Solid Edge part; units mm, degrees
sketch "Sketch1" plane through (0, 0, 0) normal (0, 0, 1) x (1, 0, 0)
  line L0 (-22.225, -31.115) -> (37.465, -31.115)
  line L1 (37.465, -31.115) -> (37.465, 31.115)
  line L2 (-37.465, 31.115) -> (37.465, 31.115)
  line L3 (-37.465, -12.065) -> (-37.465, 31.115)
  line L4 (-37.465, -12.065) -> (-22.225, -27.305)
  line L5 (-22.225, -27.305) -> (-22.225, -31.115)
  circle A0 centre (-26.035, -16.03) radius 1.5625
  circle A1 centre (-32.385, 27.15) radius 1.5625
  circle A2 centre (32.385, 6.83) radius 1.5625
extrude "Protrusion1" add sketch "Sketch1" along normal blind 1.5
sketch "Sketch2" plane through (0, 0, 1.5) normal (0, 0, 1) x (1, 0, 0)
  line L0 (4.1366, -24.673) -> (4.1366, 20.327)
  line L1 (4.1366, 20.327) -> (-13.8634, 20.327)
  line L2 (-13.8634, 20.327) -> (-13.8634, -24.673)
  line L3 (-13.8634, -24.673) -> (4.1366, -24.673)
extrude "ExtrudedProtrusion_2" add sketch "Sketch2" along normal blind 18
sketch "Sketch3" plane through (-4.8634, -24.673, 10.5) normal (0, -1, 0) x (1, 0, 0)
  line L0 (-7.5, -9) -> (-7.5, 6.914)
  line L1 (-7.5, 6.914) -> (7.5, 6.914)
  line L2 (7.5, 6.914) -> (7.5, -9)
  line L3 (7.5, -9) -> (-7.5, -9)
extrude "ExtrudedCutout_1" cut sketch "Sketch3" against normal blind 56
sketch "Sketch4" plane through (-4.8634, -24.673, 10.5) normal (0, -1, 0) x (1, 0, 0)
  line L0 (10, 6.914) -> (-10, 6.914)
  line L1 (-10, 6.914) -> (-10, 9)
  line L2 (-10, 9) -> (10, 9)
  line L3 (10, 9) -> (10, 6.914)
extrude "ExtrudedProtrusion_3" add sketch "Sketch4" against normal blind 45
sketch "Sketch5" plane through (-4.8634, 20.327, 10.5) normal (0, 1, 0) x (-1, 0, 0)
  line L0 (3.5, 12.5) -> (-3.5, 12.5)
  arc A0 (-3.5, 12.5) -> (-4, 12) centre (-3.5, 12) ccw
  line L1 (-4, 12) -> (-4, 11)
  arc A1 (-4, 11) -> (-3.5, 10.5) centre (-3.5, 11) ccw
  arc A2 (-3.5, 10.5) -> (-3, 10) centre (-3.5, 10) cw
  line L2 (-3, 10) -> (-3, 9.5)
  arc A3 (-3, 9.5) -> (-2.5, 9) centre (-2.5, 9.5) ccw
  line L3 (-2.5, 9) -> (2.5, 9)
  arc A4 (2.5, 9) -> (3, 9.5) centre (2.5, 9.5) ccw
  line L4 (3, 9.5) -> (3, 10)
  arc A5 (3, 10) -> (3.5, 10.5) centre (3.5, 10) cw
  arc A6 (4, 11) -> (3.5, 10.5) centre (3.5, 11) cw
  line L5 (4, 11) -> (4, 12)
  arc A7 (3.5, 12.5) -> (4, 12) centre (3.5, 12) cw
extrude "ExtrudedProtrusion_4" add sketch "Sketch5" along normal mid plane 8
Verification items for the finished model (mm, model axes). A direction names the side the tool comes from. Coordinates: 2 decimals unless noted, no trailing zeros. Loops run counter-clockwise (first coordinate to the right, second up) from the corner with the lowest first, then second, coordinate; pieces in that order, holes last. Notation, with made-up numbers: (42.25, 32.5) -> (62.25, 32.5) arc R21 cw to (62.25, 44.5) -> close; hole circle Ø11 at (51.25, -8.5). An arc over 180 degrees is marked (long way). Answer in a Markdown table with one row per item. Add a question column.
1. Section check C-C, the plane y = 15.5. Enter the section's corners in (x, z) (3 decimals), then the cut area to 3 significant figures.
2. Section check D-D, the plane x = 17. Enter the section's corners in (y, z) (3 decimals).
3. Material ranges on probe 1 along X at (y, z) = (-12, 13.25); probe 2 along Z at (x, y) = (-6, -19); probe 3 along Z at (x, y) = (14, 24.5), recorded low to high. Write a range as [from, to].
4. Section check A-A, the plane y = 6.83. Enter the section's corners in (x, z) (1 decimal).
5. Section check B-B, the plane y = 27.15. Enter the section's corners in (x, z) (1 decimal).
6. Access from +Z, -Z, +X, -X, +Y, -Y to the whole of each face (thin tool, end or side, straight path). Record for faces 1 (the face through (2.637, -2, 10)), 2 (the face through (-4, -24.673, 18)), 3 (the face through (4.137, -2, 9)), 4 (the face through (-13.863, -2, 9)).
7. Draft check along X on faces 5 (the face through (5.137, -2, 18)), 6 (the face through (-5, 22, 19.5)), 7 (the face through (-5, -2, 17.414)), 8 (the face through (-27.596, -16.099, 0.74)). Enter one of: +X half, -X half, draft (parallel to the pull), parting line (faces both ways), or undercut.
8. Depth check by flat-ended pin: P1, Ø2, axis at x = 27.5, y = 20, coming from the +Z side; P2, Ø3, axis at y = 0, z = 5.5, coming from the +X side; P3, Ø6, axis at x = -11, y = -24.5, coming from the +Z side; P4, Ø3, axis at x = -21, y = -23.5, coming from the -Z side. Enter the tip coordinate at first touch or a pass-through.
Derived:
| question | item | result |
|---|---|---|
| 1 | outline | (-37.465, 0) -> (37.465, 0) -> (37.465, 1.5) -> (4.137, 1.5) -> (4.137, 17.414) -> (5.137, 17.414) -> (5.137, 19.5) -> (-14.863, 19.5) -> (-14.863, 17.414) -> (-13.863, 17.414) -> (-13.863, 1.5) -> (-37.465, 1.5) -> close; hole (-12.363, 1.5) -> (2.637, 1.5) -> (2.637, 17.414) -> (-12.363, 17.414) -> close |
| 1 | area | 202 mm² |
| 2 | outline | (-31.115, 0) -> (31.115, 0) -> (31.115, 1.5) -> (-31.115, 1.5) -> close |
| 3 | probe 1 | x = [-13.86, -12.36], [2.64, 4.14] |
| 3 | probe 2 | z = [0, 1.5], [17.41, 19.5] |
| 3 | probe 3 | z = [0, 1.5] |
| 4 | outline | (-37.5, 0) -> (30.8, 0) -> (30.8, 1.5) -> (4.1, 1.5) -> (4.1, 17.4) -> (5.1, 17.4) -> (5.1, 19.5) -> (-14.9, 19.5) -> (-14.9, 17.4) -> (-13.9, 17.4) -> (-13.9, 1.5) -> (-37.5, 1.5) -> close; (33.9, 0) -> (37.5, 0) -> (37.5, 1.5) -> (33.9, 1.5) -> close; hole (-12.4, 1.5) -> (2.6, 1.5) -> (2.6, 17.4) -> (-12.4, 17.4) -> close |
| 5 | outline | (-37.5, 0) -> (-33.9, 0) -> (-33.9, 1.5) -> (-37.5, 1.5) -> close; (-30.8, 0) -> (37.5, 0) -> (37.5, 1.5) -> (-30.8, 1.5) -> close |
| 6 | face 1 | +Y, -Y |
| 6 | face 2 | +Z, +X, -X, -Y |
| 6 | face 3 | +X, +Y, -Y |
| 6 | face 4 | -X, +Y, -Y |
| 7 | face 5 | +X half |
| 7 | face 6 | draft |
| 7 | face 7 | undercut |
| 7 | face 8 | undercut |
| 8 | P1 | stops at z = 1.5 |
| 8 | P2 | stops at x = 4.14 |
| 8 | P3 | stops at z = 19.5 |
| 8 | P4 | stops at z = 0 |
